Check sheet for the modelled part. Datum: model origin and axes. Units: mm. Face numbers are marked on the shaded views. A direction names the side the tool comes from. Coordinates: 2 decimals unless noted, no trailing zeros. Loops run counter-clockwise (first coordinate to the right, second up) from the corner with the lowest first, then second, coordinate; pieces in that order, holes last. Notation, with made-up numbers: (64, -13) - (75, -13) arc R26 ccw to (75, 1) - close; hole circle Ø3 at (10, 59). An arc over 180 degrees is marked (long way). Write each question's results on one line, items separated by ' | '. Start each with the question number.
1. Tool access check on the marked faces 5, 6 and 7. Record the directions out of +Z, -Z, +X, -X, +Y, -Y that give a thin tool (end or side, any length) a straight path to the whole face; none if there is none.
2. Cross-section at C-C (x = -6). Record the cut outline in (y, z), and give its area (3 significant figures).
3. Draft check along X on the marked faces 1, 2, 3 and 4. Enter one of: released by +X, released by -X, zero draft, split by the parting line, or undercut.
4. Cross-section at A-A (x = -30). Record the cut outline in (y, z).
5. Gauge pin test, flat ends, axial feed: P1, Ø1.3, axis at x = -38, z = -23.5, coming from the +Y side; P2, Ø2, axis at y = 13.5, z = -44.5, coming from the -X side; P3, Ø2, axis at y = 5, z = 4.5, coming from the -X side; P4, Ø5, axis at x = -18, y = 14, coming from the +Z side. Record the tip position at first contact, or that the pin passes through.
6. Cross-section at D-D (y = 12). Record the cut outline in (x, z), and give its area (3 significant figures).
7. Thickness scan on line 1 (Z direction, x = -30.4, y = 15.6); line 2 (Y direction, x = -30.45, z = -45.1); line 3 (Z direction, x = -39, y = 9.9). Record the ranges inside material, lowest first. Write a range as [from, to].
8. Cross-section at B-B (y = 4.2). Record the cut outline in (x, z).
Autodesk Inventor part; units mm, degrees
ref_plane "Plano de trabajo1" through (-28.55, 0, -20.25) normal (0, 0, 1) x (1, 0, 0)
ref_plane "YZ Plane" through (0, 0, 0) normal (1, 0, 0) x (0, 1, 0)
ref_plane "XZ Plane" through (0, 0, 0) normal (0, 1, 0) x (-1, 0, 0)
sketch "Boceto1" plane through (0, 0, 0) normal (0, 1, 0) x (-1, 0, 0)
  line L0 (0, 0) -> (36.8, 0)
  line L1 (36.8, 0) -> (36.8, -40.5)
  line L2 (36.8, -40.5) -> (0, -40.5)
  line L3 (0, -40.5) -> (0, 0)
  line L4 (0, -40.5) -> (28.55, -40.5)
  line L5 (28.55, -40.5) -> (28.55, -47.65)
  line L6 (28.55, -47.65) -> (31.05, -47.65)
  line L7 (31.05, -47.65) -> (31.05, -40.5)
  line L8 (28.55, 0) -> (28.55, 7.15)
  line L9 (28.55, 7.15) -> (31.05, 7.15)
  line L10 (31.05, 7.15) -> (31.05, 0)
  dimension "d0" = 36.8
  dimension "d1" = 40.5
  dimension "d2" = 28.55
  dimension "d3" = 7.15
  dimension "d4" = 2.5
  dimension "d5" = 7.15
  dimension "d6" = 2.5
extrude "Extrusión1" add sketch "Boceto1" along normal blind 19.8
sketch "Boceto2" plane through (-36.8, 0, -40.5) normal (-1, 0, 0) x (0, 0, 1)
  line L0 (0, 0) -> (40.5, 0)
  line L1 (40.5, 0) -> (40.5, 19.8)
  line L2 (0, 19.8) -> (40.5, 19.8)
  line L3 (0, 0) -> (0, 19.8)
  line L4 (0, 0) -> (5.65, 0)
  line L5 (40.5, 18.85) -> (40.5, 0.95)
  line L6 (26.3683, 0.95) -> (5.65, 0.95)
  line L7 (40.5, 0) -> (40.5, 19.8)
  line L8 (40.5, 9.9) -> (30.6, 9.9)
  arc A0 (26.3683, 0.95) -> (26.3683, 18.85) centre (30.6, 9.9) ccw
  arc A1 (5.65, 14.48) -> (5.65, 5.32) centre (9.7412, 9.9) ccw
  line L9 (5.65, 18.85) -> (26.3683, 18.85)
  line L10 (5.65, 0.95) -> (5.65, 5.32)
  line L11 (5.65, 14.48) -> (5.65, 18.85)
  line L12 (5.65, 0.95) -> (5.65, 5.32)
  line L13 (5.65, 14.48) -> (5.65, 18.85)
  point P0 (5.65, 0.95)
  dimension "d11" = 17.9
  dimension "d12" = 9.9
extrude "Extrusión2" add sketch "Boceto2" along normal blind 2.52 contours A0 L6 L10 A1 L11 L9
sketch "Boceto3" plane through (-39.32, 0, -40.5) normal (-1, 0, 0) x (0, 0, 1)
  arc A0 (26.3683, 0.95) -> (26.3683, 18.85) centre (30.6, 9.9) ccw
  line L0 (26.3683, 18.85) -> (5.65, 18.85)
  line L1 (5.65, 18.85) -> (5.65, 14.48)
  arc A1 (5.65, 14.48) -> (5.65, 5.32) centre (9.7412, 9.9) ccw
  line L2 (5.65, 5.32) -> (5.65, 0.95)
  line L3 (5.65, 0.95) -> (26.3683, 0.95)
  circle A2 centre (30.6, 9.9) radius 6.575
  point P0 (40.5, 0)
  dimension "d18" = 13.15
extrude "Extrusión3" add sketch "Boceto3" along normal blind 2.15 contours A2
sketch "Boceto4" plane through (-41.47, 9.9, -9.9) normal (-1, 0, 0) x (0, 0, 1)
  circle A0 centre (0, 0) radius 6.575
  circle A1 centre (0, 0) radius 2.9
  point P0 (9.9, -9.9)
  dimension "d21" = 5.8
extrude "Extrusión4" add sketch "Boceto4" along normal blind 3.9 contours A1
sketch "Boceto5" plane through (-45.37, 9.9, -9.9) normal (-1, 0, 0) x (0, 0, 1)
  circle A0 centre (0, 0) radius 2.9
  point P0 (9.9, -9.9)
hole "Agujero1" at (-45.37, 9.9, -9.9) direction (1, 0, 0) diameter 2.6 depth 10 tip angle 118
sketch "Boceto6" plane through (-28.55, 0, 0) normal (0, 0, 1) x (1, 0, 0)
  line L0 (0, 0) -> (28.55, 0)
  line L1 (28.55, 0) -> (28.55, 19.8)
  line L2 (0, 19.8) -> (28.55, 19.8)
  line L3 (0, 0) -> (0, 19.8)
  line L4 (21, 9.9) -> (21, 12.8)
  line L5 (21, 12.8) -> (24.8, 12.8)
  line L6 (24.8, 12.8) -> (24.8, 7)
  line L7 (24.8, 7) -> (21, 7)
  line L8 (21, 7) -> (21, 12.8)
  line L9 (24.8, 12.8) -> (28.55, 12.8)
  dimension "d34" = 2.9
  dimension "d35" = 5.8
extrude "Extrusión5" add sketch "Boceto6" along normal blind 3.9 contours L6 L7 L8 L4 L5
sketch "Boceto7" plane through (-31.05, 0, 0) normal (-1, 0, 0) x (0, 0, 1)
  line L0 (0, 0) -> (7.15, 0)
  line L1 (7.15, 0) -> (7.15, 19.8)
  line L2 (0, 19.8) -> (7.15, 19.8)
  line L3 (0, 0) -> (0, 19.8)
  line L4 (0, 0) -> (2.26, 0)
  line L5 (2.26, 0) -> (2.26, 19.8)
  line L6 (7.15, 9.9) -> (0, 9.9)
  line L7 (7.15, 10.4) -> (0, 10.4)
  line L8 (7.15, 9.4) -> (0, 9.4)
  point P0 (0, 0)
  point P1 (0, 10.4)
  point P2 (0, 9.4)
  dimension "d38" = 2.26
  dimension "d39" = 0.5
  dimension "d40" = 0.5
extrude "Extrusión6" add sketch "Boceto7" along normal blind 1.35 contours L3 L6 L5 L8 | L5 L6 L1 L8 | L3 L7 L5 L6 | L5 L7 L1 L6
chamfer "Chaflán1" distance 6 distance2 1.35 1 edges at (-32.4, 9.9, 7.15) measured on face at (-32.4, 9.7333, 4.7667)
fillet "Empalme1" radius 2 2 edges at (-29.8, 0, 7.15) (-29.8, 19.8, 7.15)
sketch "Boceto8" plane through (-31.05, 0, 0) normal (-1, 0, 0) x (0, 0, 1)
  arc A0 (5.15, 0) -> (7.15, 2) centre (5.15, 2) ccw
  line L0 (7.15, 2) -> (7.15, 9.4)
  line L1 (7.15, 9.4) -> (0, 9.4)
  line L2 (0, 0) -> (0, 9.4)
  line L3 (0, 0) -> (5.15, 0)
  line L4 (3.575, 0) -> (3.575, 2)
  line L5 (3.575, 2) -> (3.575, 6.4)
  line L6 (0, 0) -> (2.4, 0)
  line L7 (2.4, 0) -> (2.4, 4.2)
  line L8 (2.4, 4.2) -> (4.6, 4.2)
  circle A1 centre (4.6, 4.2) radius 2.2
  arc A2 (7.15, 17.8) -> (5.15, 19.8) centre (5.15, 17.8) ccw
  line L9 (0, 19.8) -> (5.15, 19.8)
  line L10 (0, 10.4) -> (0, 19.8)
  line L11 (0, 10.4) -> (7.15, 10.4)
  line L12 (7.15, 10.4) -> (7.15, 17.8)
  line L13 (4.6, 4.2) -> (4.6, 19.8)
  line L14 (4.6, 19.8) -> (4.6, 15.6)
  circle A3 centre (4.6, 15.6) radius 2.2
  point P0 (0, 0)
  dimension "d47" = 2
  dimension "d48" = 4.4
  dimension "d49" = 2.4
  dimension "d50" = 2.2
  dimension "d58" = 4.2
  dimension "d59" = 4.4
hole "Agujero2" at (-31.05, 4.2, 4.6) at (-31.05, 15.6, 4.6) direction (1, 0, 0) diameter 4.4 depth 10 tip angle 118
ref_plane "Plano de trabajo1" through (-28.55, 0, -20.25) normal (0, 0, 1) x (1, 0, 0)
mirror "Simetría1" about plane through (-28.55, 0, -20.25) normal (0, 0, 1) of "Extrusión6", "Agujero2"
chamfer "Chaflán2" distance 6 distance2 1.35 1 edges at (-32.4, 9.9, -47.65) measured on face at (-32.4, 9.7333, -45.2667)
fillet "Empalme2" radius 2 2 edges at (-29.8, 0, -47.65) (-29.8, 19.8, -47.65)
ref_plane "Plano de trabajo2" through (0, 9.9, 0) normal (0, -1, 0) x (1, 0, 0)
properties part number "ServoMotor"
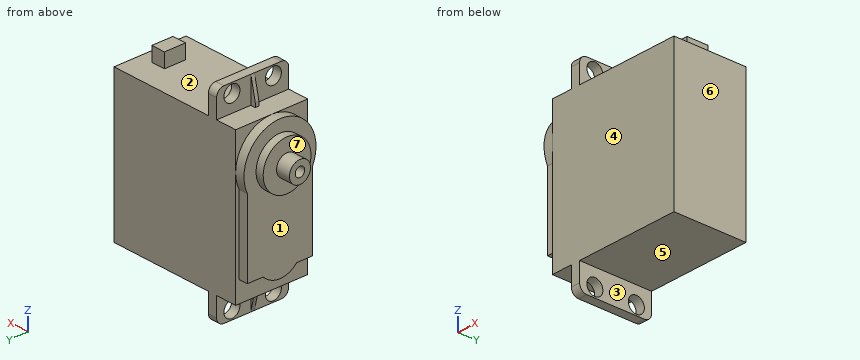
Established:
1) face 5: -Z, +X, +Y, -Y | face 6: +Z, -Z, +X, +Y, -Y | face 7: -X
2) outline: (0, -40.5) - (19.8, -40.5) - (19.8, 0) - (12.8, 0) - (12.8, 3.9) - (7, 3.9) - (7, 0) - (0, 0) - close | area: 825 mm^2
3) face 1: released by -X | face 2: undercut | face 3: released by +X | face 4: zero draft
4) outline: (0, -45.65) arc R2 ccw to (2, -47.65) - (17.8, -47.65) arc R2 ccw to (19.8, -45.65) - (19.8, 5.15) arc R2 ccw to (17.8, 7.15) - (2, 7.15) arc R2 ccw to (0, 5.15) - close; hole circle Ø4.4 at (4.2, -45.1); hole circle Ø4.4 at (4.2, 4.6); hole circle Ø4.4 at (15.6, -45.1); hole circle Ø4.4 at (15.6, 4.6)
5) P1: y = 18.85 | P2: x = -31.05 | P3: through | P4: z = 0
6) outline: (-45.37, -11.9) - (-41.47, -11.9) - (-41.47, -16.13) - (-39.32, -16.13) - (-39.32, -36.53) - (-36.8, -36.53) - (-36.8, -40.5) - (-31.05, -40.5) - (-31.05, -47.65) - (-28.55, -47.65) - (-28.55, -40.5) - (0, -40.5) - (0, 0) - (-3.75, 0) - (-3.75, 3.9) - (-7.55, 3.9) - (-7.55, 0) - (-28.55, 0) - (-28.55, 7.15) - (-31.05, 7.15) - (-31.05, 0) - (-36.8, 0) - (-36.8, -0.23) - (-39.32, -0.23) - (-39.32, -3.67) - (-41.47, -3.67) - (-41.47, -7.9) - (-45.37, -7.9) - close | area: 1,670 mm^2
7) line 1: [-47.65, -47.3], [-42.9, 2.4], [6.8, 7.15] | line 2: [0, 2], [6.4, 13.4], [17.8, 19.8] | line 3: [-36.9, -11.2], [-8.6, 0]
8) outline: (-41.47, -13.18) - (-39.32, -13.18) - (-39.32, -34.85) - (-36.8, -34.85) - (-36.8, -40.5) - (-31.05, -40.5) - (-31.05, -42.9) - (-28.55, -42.9) - (-28.55, -40.5) - (0, -40.5) - (0, 0) - (-28.55, 0) - (-28.55, 2.4) - (-31.05, 2.4) - (-31.05, 0) - (-36.8, 0) - (-36.8, -1.81) - (-39.32, -1.81) - (-39.32, -6.62) - (-41.47, -6.62) - close; (-31.05, -47.65) - (-28.55, -47.65) - (-28.55, -47.3) - (-31.05, -47.3) - close; (-31.05, 6.8) - (-28.55, 6.8) - (-28.55, 7.15) - (-31.05, 7.15) - close
